```python
from build123d import *

# Parameters (mm, degrees)
SKETCH1_R              = 75
SKETCH1_W              = 60
SKETCH1_H              = 60
BOSS_EXTRUDE1_DEPTH    = 20
SKETCH1_2_W            = 60
SKETCH1_2_H            = 60
BOSS_EXTRUDE2_DEPTH    = 360
CUT_EXTRUDE1_DEPTH     = 383.426463519
CUT_EXTRUDE2_START     = -60
CUT_EXTRUDE2_OUTLINE_R = 20
CUT_EXTRUDE2_DEPTH     = 60


# Read off the part's stored shape, not the designer's step: Cut-Extrude2
with BuildPart() as part:
    # Sketch1 → Boss-Extrude1 (new body)
    with BuildSketch(Plane(origin=(0, 0, 0), x_dir=(1, 0, 0), z_dir=(0, 1, 0))):
        with Locations(Location((0, 0, 0), (0, 0, 270))):
            Circle(SKETCH1_R)
        Rectangle(SKETCH1_W, SKETCH1_H, mode=Mode.SUBTRACT)
    extrude(amount=BOSS_EXTRUDE1_DEPTH)

    # Sketch1_2 → Boss-Extrude2 (add)
    with BuildSketch(Plane(origin=(0, 0, 0), x_dir=(1, 0, 0), z_dir=(0, 1, 0))):
        Rectangle(SKETCH1_2_W, SKETCH1_2_H)
    extrude(amount=BOSS_EXTRUDE2_DEPTH)

    # Sketch2 → Cut-Extrude1 (cut, through all)
    with BuildSketch(Plane(origin=(30, 0, 0), x_dir=(0, 0, -1), z_dir=(1, 0, 0))):
        with BuildLine():
            Line((-20, 360), (20, 360))
            Line((20, 360), (20, 180))
            ThreePointArc((20, 180), (0, 160), (-20, 180))
            Line((-20, 180), (-20, 360))
        make_face()
    extrude(amount=-CUT_EXTRUDE1_DEPTH, mode=Mode.SUBTRACT)

    # Cut-Extrude2 outline → Cut-Extrude2 (cut)
    with BuildSketch(Plane.XY.offset(30).offset(CUT_EXTRUDE2_START)):
        with Locations((0, 330)):
            Circle(CUT_EXTRUDE2_OUTLINE_R)
        with BuildLine():
            ThreePointArc((-30, 330), (-21.213203436, 351.213203436), (0, 360))
            Line((0, 360), (-30, 360))
            Line((-30, 360), (-30, 330))
        make_face()
        with BuildLine():
            ThreePointArc((0, 360), (21.213203436, 351.213203436), (30, 330))
            Line((30, 330), (30, 360))
            Line((30, 360), (0, 360))
        make_face()
    extrude(amount=CUT_EXTRUDE2_DEPTH, mode=Mode.SUBTRACT)


solid = part.part
```
Input: part model. Units: mm. Frame: model coordinates. A direction names the side the tool comes from. Round coordinates to 2 decimals unless told otherwise and drop trailing zeros. Loops run counter-clockwise (first coordinate to the right, second up) from the corner with the lowest first, then second, coordinate; pieces in that order, holes last. Notation, with made-up numbers: (24.25, -33) -> (55.25, -33) arc R27 cw to (55.25, -15) -> close; hole circle Ø8 at (-7, 75). An arc over 180 degrees is marked (long way). One line per item, written item: value.
(1) Mould query, pull axis Y, two halves, no side actions, for faces 1 (the face through (0, 188, 30)), 2 (the face through (1, 0, -1)), 3 (the face through (-4.336, 310.476, -25.07)). Classes: pulls with the +Y half, pulls with the -Y half, needs draft (parallel to the pull), parting line crosses it, or undercut.
Geometry check:
face 1: needs draft
face 2: pulls with the -Y half
face 3: undercut
(2) Material intervals for line 1 (X direction, y = 330, z = 23); line 2 (Y direction, x = 13, z = -43.5), sorted ascending. Write a range as [from, to].
Geometry check:
line 1: [-30, -20], [20, 30]
line 2: [0, 20]
(3) Set-up query: faces 4 (the face through (0, 271, -20)), 5 (the face through (-30, 138, 0)), 6 (the face through (30, 138, 0)), 7 (the face through (0, 188, -30)). Return all of +Z, -Z, +X, -X, +Y, -Y with unobstructed straight access to the full face (end or side cutting, diameter ignored); none if empty.
Geometry check:
face 4: +X, -X, +Y
face 5: +Z, -Z, -X, +Y
face 6: +Z, -Z, +X, +Y
face 7: -Z, +X, -X, +Y
(4) Pin query (flat end, axial travel): pin 1 (18 mm diameter, centred on y = 167, z = -4, fed in from +X); pin 2 (5 mm diameter, centred on x = -17, y = 196, fed in from -Z); pin 3 (1.5 mm diameter, centred on x = 32, y = 236, fed in from +Z); pin 4 (5 mm diameter, centred on x = 25, y = 263, fed in from +Z). Return the tip coordinate at first contact, or that it passes through.
Geometry check:
pin 1: x = 30
pin 2: z = -30
pin 3: through
pin 4: z = 30
(5) Section A-A (y = 186). Return the cut outline in (x, z), plus the area to 3 significant figures.
Geometry check:
outline: (-30, -30) -> (30, -30) -> (30, -20) -> (-30, -20) -> close; (-30, 20) -> (30, 20) -> (30, 30) -> (-30, 30) -> close
area: 1,200 mm2
(6) Section D-D (x = 45). Return the cut outline in (y, z), plus the area to 3 significant figures.
Geometry check:
outline: (0, -60) -> (20, -60) -> (20, 60) -> (0, 60) -> close
area: 2,400 mm2
(7) Section C-C (y = 334). Return the cut outline in (x, z).
Geometry check:
outline: (-29.73, -30) -> (-19.6, -30) -> (-19.6, -20) -> (-29.73, -20) -> close; (-29.73, 20) -> (-19.6, 20) -> (-19.6, 30) -> (-29.73, 30) -> close; (19.6, -30) -> (29.73, -30) -> (29.73, -20) -> (19.6, -20) -> close; (19.6, 20) -> (29.73, 20) -> (29.73, 30) -> (19.6, 30) -> close
(8) Section B-B (x = -15.5). Return the cut outline in (y, z).
Geometry check:
outline: (0, -73.38) -> (20, -73.38) -> (20, -30) -> (317.36, -30) -> (317.36, -20) -> (180, -20) arc R20 cw to (180, 20) -> (317.36, 20) -> (317.36, 30) -> (20, 30) -> (20, 73.38) -> (0, 73.38) -> close; (342.64, -30) -> (355.69, -30) -> (355.69, -20) -> (342.64, -20) -> close; (342.64, 20) -> (355.69, 20) -> (355.69, 30) -> (342.64, 30) -> close
